Model file for the job. Use its own axes, mm. A direction names the side the tool comes from. Coordinates: 2 decimals unless noted, no trailing zeros. Write each loop counter-clockwise with the first axis right and the second up, starting at its lowest first coordinate (ties: lowest second). Pieces come first, ordered by that corner, then holes. Notation, with made-up numbers: M -38.5,48.25 L -1.5,48.25 A15 ccw -1.5,72.25 Z; hole C -36.75,87 d1. An arc over 180 degrees is marked long. One line per question, with ' | ' between items. Start each with the question number.
(1) Tool access for faces 4 (the face through (10, 42, 79.287)), 5 (the face through (2, 40, 49)), 6 (the face through (9.909, 36.746, 93.26)), 7 (the face through (20, 42, 49)), 8 (the face through (10, 50, 48)): list every direction of +Z, -Z, +X, -X, +Y, -Y with a clear straight run to the whole face (end or side of a thin tool).
(2) Cut at B-B (z = 11.5). Write the cut outline in (x, y).
(3) Cut at C-C (x = 10). Count the separate pieces of the cut face and the enclosed holes in it, plus the area to 3 significant figures.
(4) Two-plate mould, pull along Z, no slides. Class faces 1 (the face through (18, 40, 49)), 2 (the face through (10, 25, 98)), 3 (the face through (10, 0, 2)): +Z half, -Z half, draft (parallel to the pull), parting line (faces both ways), or undercut.
(5) Cut at A-A (y = 11). Write the cut outline in (x, z).
(6) Cut at D-D (z = 28.5). Write the cut outline in (x, y).
(7) Wall check: probe 1 along Y at (x, z) = (10, 95.75); probe 2 along Z at (x, y) = (3.75, 27); probe 3 along Z at (x, y) = (8.5, 44). Give the ranges that are in metal, low to high.
(8) Flat gauge pins, fed straight in: pin 1 Ø1.8 at (x, z) = (2, 42.5) entering from -Y; pin 2 Ø2 at (x, z) = (9.5, 87.5) entering from -Y; pin 3 Ø6 at (x, z) = (12.5, 61.5) entering from -Y. Where does each tip first touch, or does it go through?
from build123d import *

# Parameters (mm, degrees)
SKETCH1_W           = 20
SKETCH1_H           = 50
BOSS_EXTRUDE1_DEPTH = 5
SKETCH3_R           = 2.5
CUT_EXTRUDE5_DEPTH  = 5
SKETCH4_W           = 20
SKETCH4_H           = 10
BOSS_EXTRUDE2_DEPTH = 88
SKETCH5_W           = 20
SKETCH5_H           = 50
BOSS_EXTRUDE3_DEPTH = 5
CUT_EXTRUDE6_START  = -5
SKETCH6_R           = 2.5
CUT_EXTRUDE6_DEPTH  = 5
BOSS_EXTRUDE4_DEPTH = 20
FILLET1_R           = 15
SHELL2_START        = 3.5
SHELL2_DEPTH        = 13


# Read off the part's stored shape, not the designer's step: Shell2
with BuildPart() as part:
    # Sketch1 → Boss-Extrude1 (new body)
    with BuildSketch(Plane.XY):
        with Locations((10, 25)):
            Rectangle(SKETCH1_W, SKETCH1_H)
    extrude(amount=BOSS_EXTRUDE1_DEPTH)

    # Sketch3 → Cut-Extrude5 (cut)
    with BuildSketch(Plane(origin=(0, 0, 0), x_dir=(-1, 0, 0), z_dir=(0, 0, -1))):
        with Locations((-10, 7.5)):
            Circle(SKETCH3_R)
        with Locations((-10, 20)):
            Circle(SKETCH3_R)
    extrude(amount=-CUT_EXTRUDE5_DEPTH, mode=Mode.SUBTRACT)

    # Sketch4 → Boss-Extrude2 (add)
    with BuildSketch(Plane.XY.offset(5)):
        with Locations((10, 45)):
            Rectangle(SKETCH4_W, SKETCH4_H)
    extrude(amount=BOSS_EXTRUDE2_DEPTH)

    # Sketch5 → Boss-Extrude3 (add)
    with BuildSketch(Plane.XY.offset(93)):
        with Locations((10, 25)):
            Rectangle(SKETCH5_W, SKETCH5_H)
    extrude(amount=BOSS_EXTRUDE3_DEPTH)

    # Sketch6 → Cut-Extrude6 (cut)
    with BuildSketch(Plane.XY.offset(98).offset(CUT_EXTRUDE6_START)):
        with Locations(Location((10, 7.5, 0), (0, 0, 180))):
            Circle(SKETCH6_R)
        with Locations(Location((10, 20, 0), (0, 0, 180))):
            Circle(SKETCH6_R)
    extrude(amount=CUT_EXTRUDE6_DEPTH, mode=Mode.SUBTRACT)

    # Sketch7 → Boss-Extrude4 (add)
    with BuildSketch(Plane(origin=(20, 0, 0), x_dir=(0, 0, -1), z_dir=(1, 0, 0))):
        Polygon((-93, 40), (-85.5, 40), (-93, 32.5), align=None)
        Polygon((-12.5, 40), (-5, 40), (-5, 32.5), align=None)
    extrude(amount=-BOSS_EXTRUDE4_DEPTH)

    # Fillet1
    # the kernel refuses this fillet: 15 mm, written as the material it adds along each edge
    with BuildSketch(Plane(origin=(20, 32.5, 5), x_dir=(0, -1, 0), z_dir=(-1, 0, 0)), Plane(origin=(20, 40, 85.5), x_dir=(0, 0, -1), z_dir=(-1, 0, 0))) as fillet1_piece_1:
        with BuildLine():
            CenterArc((FILLET1_R * 0.414213562373, FILLET1_R), FILLET1_R, 225, 45)
            Line((-FILLET1_R * 0.292893218813, FILLET1_R * 0.292893218813), (0, 0))
            Line((0, 0), (FILLET1_R * 0.414213562373, 0))
        make_face()
    extrude(amount=20)
    with BuildSketch(Plane(origin=(20, 40, 12.5), x_dir=(0, 0, 1), z_dir=(-1, 0, 0)), Plane(origin=(20, 32.5, 93), x_dir=(0, -1, 0), z_dir=(-1, 0, 0))) as fillet1_piece_2:
        with BuildLine():
            CenterArc((FILLET1_R * 0.414213562373, -FILLET1_R), FILLET1_R, 90, 45)
            Line((-FILLET1_R * 0.292893218813, -FILLET1_R * 0.292893218813), (0, 0))
            Line((0, 0), (FILLET1_R * 0.414213562373, 0))
        make_face()
    extrude(amount=20)

    # Shell2 outline → Shell2 (cut)
    with BuildSketch(Plane.YZ.offset(SHELL2_START)):
        with BuildLine():
            ThreePointArc((38.709041728, 91.709041728), (42.260754212, 85.943850268), (43.5, 79.286796564))
            Line((43.5, 79.286796564), (40, 79.286796564))
            Line((40, 79.286796564), (40, 18.713203436))
            Line((40, 18.713203436), (43.5, 18.713203436))
            ThreePointArc((43.5, 18.713203436), (42.260754212, 12.056149732), (38.709041728, 6.290958272))
            ThreePointArc((38.709041728, 6.290958272), (36.774474362, 4.759966719), (34.65339683, 3.5))
            Line((34.65339683, 3.5), (46.5, 3.5))
            Line((46.5, 3.5), (46.5, 94.5))
            Line((46.5, 94.5), (34.65339683, 94.5))
            ThreePointArc((34.65339683, 94.5), (36.774474362, 93.240033281), (38.709041728, 91.709041728))
        make_face()
    extrude(amount=SHELL2_DEPTH, mode=Mode.SUBTRACT)


solid = part.part
Filled in:
1) face 4: -Y | face 5: +X, -X, -Y | face 6: none | face 7: +Z, -Z, +X, +Y, -Y | face 8: +Z, -Z, +X, -X, +Y
2) outline: M 0,38.15 L 20,38.15 L 20,50 L 0,50 Z; hole M 3.5,42.04 L 16.5,42.04 L 16.5,46.5 L 3.5,46.5 Z
3) separate pieces: 5 | enclosed holes: 0 | area: 796 mm²
4) face 1: undercut | face 2: +Z half | face 3: draft
5) outline: M 0,0 L 20,0 L 20,5 L 0,5 Z; M 0,93 L 20,93 L 20,98 L 0,98 Z
6) outline: M 0,40 L 3.5,40 L 3.5,46.5 L 16.5,46.5 L 16.5,40 L 20,40 L 20,50 L 0,50 Z
7) probe 1: 0 to 5, 10 to 17.5, 22.5 to 50 | probe 2: 0 to 5.02, 92.98 to 98 | probe 3: 0 to 3.5, 94.5 to 98
8) pin 1: y = 40 | pin 2: y = 36.84 | pin 3: y = 46.5
